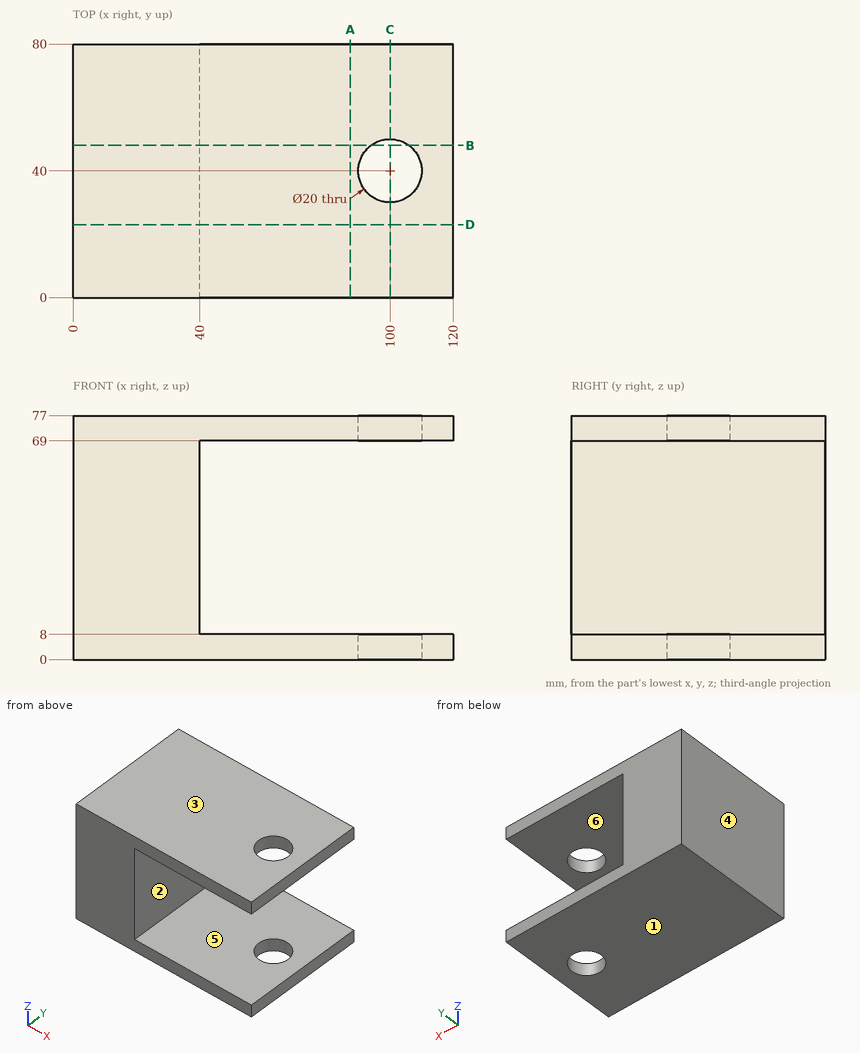
Answer from the drawing. Dimensions are ordinates in mm from the lowest x, y and z of the part. A direction names the side the tool comes from. Round coordinates to 2 decimals unless told otherwise and drop trailing zeros. Loops run counter-clockwise (first coordinate to the right, second up) from the corner with the lowest first, then second, coordinate; pieces in that order, holes last. Notation, with made-up numbers: (70, 43.25) - (76, 43.25) arc R20 cw to (76, 47.25) - close; hole circle Ø1 at (-2.75, 52.25). An arc over 180 degrees is marked (long way). Return JSON: item names as keys, results as strings. Group by question number.
1. The part is cut by section D-D on y = 23. Determine the outline of the cut face in (x, z), then the cut area to 3 significant figures.
2. Each of these flat-tipped pins is pushed along its axis until it touches: P1, Ø5, axis at x = 43.5, z = 33, coming from the +Y side; P2, Ø4, axis at y = 14, z = 25.5, coming from the +X side. Where does it stop, or does it pass through?
3. The part is cut by section A-A on x = 87.5. Determine the outline of the cut face in (y, z).
4. The mould has two halves that part along Z. Classify the marked faces 3, 4, 5 and 6: pulls with the +Z half, pulls with the -Z half, needs draft (parallel to the pull), parting line crosses it, or undercut.
5. Which of the six approach directions +Z, -Z, +X, -X, +Y, -Y give full straight-line access (tool end or side, diameter ignored) to the marked faces 1 and 2?
6. The part is cut by section B-B on y = 48. Determine the outline of the cut face in (x, z).
7. The part is cut by section C-C on x = 100. Determine the outline of the cut face in (y, z).
8. Consider probe 1 along Z at (x, y) = (65.5, 14); probe 2 along Y at (x, z) = (100, 72); probe 3 along X at (y, z) = (71, 41). Determine where each line is inside the solid, lowest interval first.
Resolved:
{
 "1": {"outline": "(0, 0) - (120, 0) - (120, 8) - (40, 8) - (40, 69) - (120, 69) - (120, 77) - (0, 77) - close", "area": "4,360 mm²"},
 "2": {"P1": "passes through", "P2": "stops at x = 40"},
 "3": {"outline": "(0, 0) - (80, 0) - (80, 8) - (0, 8) - close; (0, 69) - (80, 69) - (80, 77) - (0, 77) - close"},
 "4": {"face 3": "pulls with the +Z half", "face 4": "needs draft", "face 5": "undercut", "face 6": "undercut"},
 "5": {"face 1": "-Z, +X, -X, +Y, -Y", "face 2": "+X, +Y, -Y"},
 "6": {"outline": "(0, 0) - (94, 0) - (94, 8) - (40, 8) - (40, 69) - (94, 69) - (94, 77) - (0, 77) - close; (106, 0) - (120, 0) - (120, 8) - (106, 8) - close; (106, 69) - (120, 69) - (120, 77) - (106, 77) - close"},
 "7": {"outline": "(0, 0) - (30, 0) - (30, 8) - (0, 8) - close; (0, 69) - (30, 69) - (30, 77) - (0, 77) - close; (50, 0) - (80, 0) - (80, 8) - (50, 8) - close; (50, 69) - (80, 69) - (80, 77) - (50, 77) - close"},
 "8": {"probe 1": "z = 0 to 8, 69 to 77", "probe 2": "y = 0 to 30, 50 to 80", "probe 3": "x = 0 to 40"}
}
